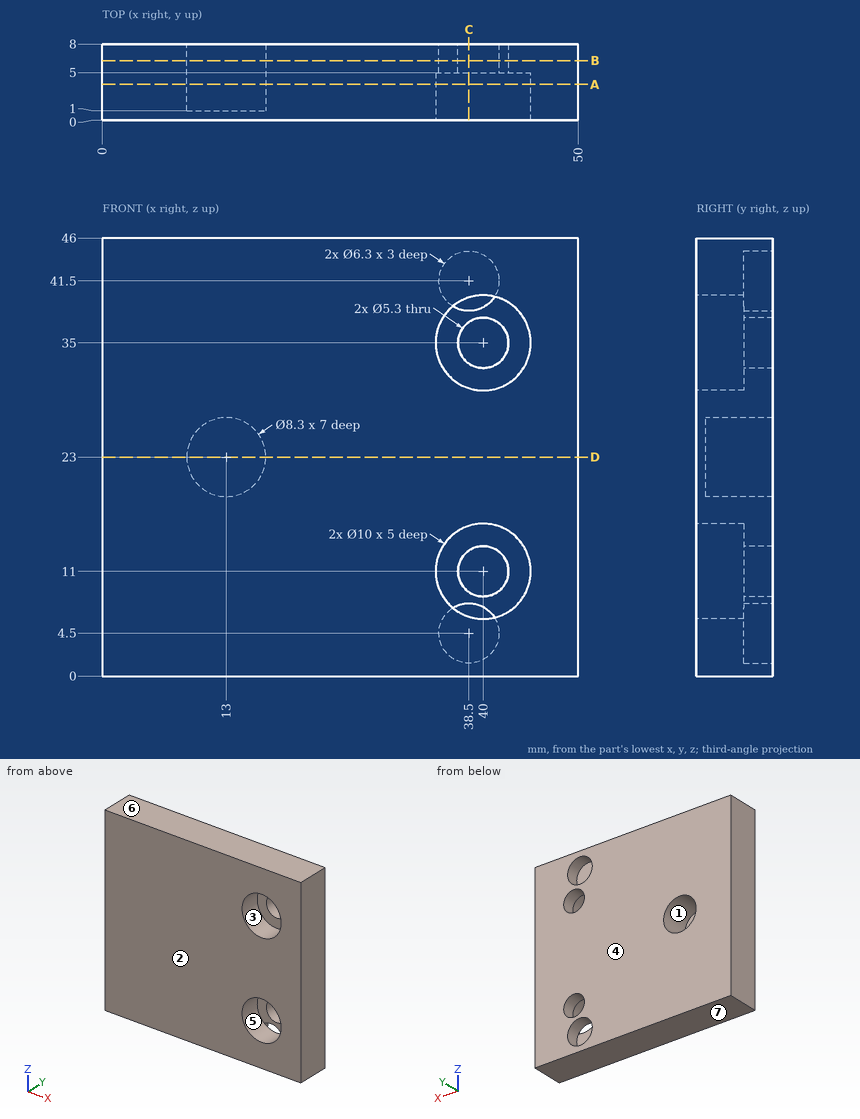
For this review, use the dimensioned drawing (mm, ordinates from the lowest corner) and the shaded views. A direction names the side the tool comes from. Coordinates: 2 decimals unless noted, no trailing zeros. Order: outer loops, then holes, each group sorted by start corner. A loop starts at its lowest first (then second) coordinate and runs counter-clockwise, first axis right, second up. Notation, with made-up numbers: M -3,-2.5 L 7,-2.5 A24 cw 7,32.5 Z; hole C 83,-13.5 d5. An arc over 180 degrees is marked long. Answer as a JSON object with one key per item and string values. Group by question number.
1) Add section A-A, the plane y = 3.75. Write out the cut boundary in (x, z), then the cut area to 3 significant figures.
2) Add section D-D, the plane z = 23. Write out the cut boundary in (x, y), then the cut area to 3 significant figures.
3) Add section C-C, the plane x = 38.5. Write out the cut boundary in (y, z).
4) For pin 1 (2.5 mm diameter, centred on x = 12.5, z = 24, fed in from +Y); pin 2 (5 mm diameter, centred on x = 40, z = 35, fed in from +Y); pin 3 (5 mm diameter, centred on x = 38.5, z = 41.5, fed in from +Y), all flat-tipped, find the tip position at first contact; note any pin that passes through.
5) Tool access review of the marked faces 1, 2 and 3: name each direction out of +Z, -Z, +X, -X, +Y, -Y from which nothing blocks a thin tool from reaching the whole face with its end or side.
6) Wall thickness on L1, parallel to X at y = 7.15, z = 4.5; L2, parallel to Z at x = 40, y = 3.55; L3, parallel to Z at x = 13, y = 3.75: over which ranges is each line inside the solid? List them lowest first.
7) Add section B-B, the plane y = 6.25. Write out the cut boundary in (x, z).
8) Mouldability with a two-part tool opening along Z and no side actions: class the marked faces 4, 5, 6 and 7 as pulls with the +Z half, pulls with the -Z half, needs draft (parallel to the pull), parting line crosses it, or undercut.
Computed values:
{
 "1": {"outline": "M 0,0 L 50,0 L 50,46 L 0,46 Z; hole C 13,23 d8.3; hole C 40,11 d10; hole C 40,35 d10", "area": "2,090 mm^2"},
 "2": {"outline": "M 0,0 L 50,0 L 50,8 L 17.15,8 L 17.15,1 L 8.85,1 L 8.85,8 L 0,8 Z", "area": "342 mm^2"},
 "3": {"outline": "M 0,0 L 8,0 L 8,1.35 L 5,1.35 L 5,6.23 L 0,6.23 Z; M 0,15.77 L 5,15.77 L 5,13.18 L 8,13.18 L 8,32.82 L 5,32.82 L 5,30.23 L 0,30.23 Z; M 0,39.77 L 5,39.77 L 5,44.65 L 8,44.65 L 8,46 L 0,46 Z; M 5,7.65 L 8,7.65 L 8,8.82 L 5,8.82 Z; M 5,37.18 L 8,37.18 L 8,38.35 L 5,38.35 Z"},
 "4": {"pin 1": "stops at y = 1", "pin 2": "passes through", "pin 3": "stops at y = 5"},
 "5": {"face 1": "+Y", "face 2": "+Z, -Z, +X, -X, -Y", "face 3": "-Y"},
 "6": {"L1": "x = 0 to 35.35, 41.65 to 50", "L2": "z = 0 to 6, 16 to 30, 40 to 46", "L3": "z = 0 to 18.85, 27.15 to 46"},
 "7": {"outline": "M 0,0 L 50,0 L 50,46 L 0,46 Z; hole C 13,23 d8.3; hole C 38.5,4.5 d6.3; hole C 38.5,41.5 d6.3; hole C 40,11 d5.3; hole C 40,35 d5.3"},
 "8": {"face 4": "needs draft", "face 5": "undercut", "face 6": "pulls with the +Z half", "face 7": "pulls with the -Z half"}
}
